The model under review builds one solid part; all positions refer to its coordinate system, in mm. Round coordinates to 2 decimals unless told otherwise and drop trailing zeros. Write each loop counter-clockwise with the first axis right and the second up, starting at its lowest first coordinate (ties: lowest second). Pieces come first, ordered by that corner, then holes. Notation, with made-up numbers: (17.25, 16.5) -> (60.25, 16.5) arc R20 cw to (60.25, 43.5) -> close; hole circle Ø5 at (60, 6). An arc over 180 degrees is marked (long way). Answer as a JSON object with one key per item and string values. Group by question number.
1) We need section A-A, the plane x = 12. Write out the cut boundary in (y, z), then the cut area to 3 significant figures.
2) We need section C-C, the plane z = 1.55. Write out the cut boundary in (x, y).
3) Insertion check: pin 1 Ø2.5 at (x, y) = (4.52, -16.03) entering from -Z; pin 2 Ø5 at (x, y) = (26, -4) entering from -Z. Each pin has a flat end and moves straight along its axis. Give the tip position at first contact, or say it passes through.
4) To check wall thickness, follow probe 1 along Y at (x, z) = (12, 1.1); probe 2 along Y at (x, z) = (5.5, 1.45); probe 3 along X at (y, z) = (-47.5, 1.75). State the ranges of each line that lie inside material, in increasing order. Write a range as [from, to].
5) Mouldability with a two-part tool opening along X and no side actions: class faces 1 (the cylindrical face through (12, -50, 1)), 2 (the cylindrical face through (0.9, -0.86, 1.01)), 3 (the flat face through (11, -20, 0)), 4 (the cylindrical face through (29.1, -0.86, 1.01)) as pulls with the +X half, pulls with the -X half, needs draft (parallel to the pull), parting line crosses it, or undercut.
6) We need section B-B, the plane y = -4. Write out the cut boundary in (x, z), then the cut area to 3 significant figures.
7) We need section D-D, the plane y = -45. Write out the cut boundary in (x, z).
from build123d import *

# Parameters (mm, degrees)
SKETCH_1_R      = 1.5
SKETCH_1_R_2    = 1.3
EXTRUDE_1_DEPTH = 2
FILLET_1_R      = 3


with BuildPart() as part:
    # 草图1 → 凸台-拉伸1 (new body)
    with BuildSketch(Plane.XY):
        Polygon((30, 0), (0, 0), (0, -52.5), (15, -52.5), (30, -10), align=None)
        with Locations((26, -4)):
            Circle(SKETCH_1_R, mode=Mode.SUBTRACT)
        with Locations((12, -48.5)):
            Circle(SKETCH_1_R, mode=Mode.SUBTRACT)
        with Locations((4.515040622, -41)):
            Circle(SKETCH_1_R_2, mode=Mode.SUBTRACT)
        with Locations((4.515040622, -16.028894545)):
            Circle(SKETCH_1_R_2, mode=Mode.SUBTRACT)
    extrude(amount=EXTRUDE_1_DEPTH)

    # 圆角1
    fillet_1_edges = [part.edges().sort_by_distance(p)[0] for p in [
        (30, -10, 1),
        (15, -52.5, 1),
        (0, -52.5, 1),
        (0, 0, 1),
        (30, 0, 1),
    ]]
    fillet(fillet_1_edges, radius=FILLET_1_R)


solid = part.part
Here are the results:
{
 "1": {"outline": "(-52.5, 0) -> (-50, 0) -> (-50, 2) -> (-52.5, 2) -> close; (-47, 0) -> (0, 0) -> (0, 2) -> (-47, 2) -> close", "area": "99.0 mm^2"},
 "2": {"outline": "(0, -49.5) arc R3 ccw to (3, -52.5) -> (12.88, -52.5) arc R3 ccw to (15.71, -50.5) -> (29.83, -10.48) arc R3 ccw to (30, -9.49) -> (30, -3) arc R3 ccw to (27, 0) -> (3, 0) arc R3 ccw to (0, -3) -> close; hole circle Ø2.6 at (4.52, -41); hole circle Ø2.6 at (4.52, -16.03); hole circle Ø3 at (12, -48.5); hole circle Ø3 at (26, -4)"},
 "3": {"pin 1": "passes through", "pin 2": "stops at z = 0"},
 "4": {"probe 1": "y = [-52.5, -50], [-47, 0]", "probe 2": "y = [-52.5, -41.85], [-40.15, -16.88], [-15.18, 0]", "probe 3": "x = [0, 10.88], [13.12, 16.76]"},
 "5": {"face 1": "undercut", "face 2": "pulls with the -X half", "face 3": "needs draft", "face 4": "pulls with the +X half"},
 "6": {"outline": "(0, 0) -> (24.5, 0) -> (24.5, 2) -> (0, 2) -> close; (27.5, 0) -> (30, 0) -> (30, 2) -> (27.5, 2) -> close", "area": "54.0 mm^2"},
 "7": {"outline": "(0, 0) -> (17.65, 0) -> (17.65, 2) -> (0, 2) -> close"}
}
